Could you check a few things on this model? Use its own coordinates, in mm. A direction names the side the tool comes from. Give positions to 0.01 mm unless a question says otherwise; leave off trailing zeros. Order: outer loops, then holes, each group sorted by start corner. A loop starts at its lowest first (then second) coordinate and runs counter-clockwise, first axis right, second up.
from build123d import *

# Parameters (mm, degrees)
BOSS_EXTRUDE1_DEPTH = 100
CUT_EXTRUDE1_DEPTH  = 8
SKETCH4_W           = 8
SKETCH4_H           = 100
BOSS_EXTRUDE2_DEPTH = 35
CUT_EXTRUDE2_DEPTH  = 8


with BuildPart() as part:
    # Sketch1 → Boss-Extrude1 (new body)
    with BuildSketch(Plane(origin=(0, 0, 0), x_dir=(1, 0, 0), z_dir=(0, 1, 0))):
        Polygon((0, 0), (8, 0), (8, 27), (40, 27), (40, 35), (0, 35), align=None)
    extrude(amount=BOSS_EXTRUDE1_DEPTH)

    # Sketch3 → Cut-Extrude1 (cut)
    with BuildSketch(Plane(origin=(0, 0, -35), x_dir=(-1, 0, 0), z_dir=(0, 0, -1))):
        with BuildLine():
            Line((-40, 20), (-35, 20))
            ThreePointArc((-35, 20), (-31.464466094, 21.464466094), (-30, 25))
            Line((-30, 25), (-30, 75))
            ThreePointArc((-30, 75), (-31.464466094, 78.535533906), (-35, 80))
            Line((-35, 80), (-40, 80))
            Line((-40, 80), (-40, 20))
        make_face()
    extrude(amount=-CUT_EXTRUDE1_DEPTH, mode=Mode.SUBTRACT)

    # Sketch4 → Boss-Extrude2 (add)
    with BuildSketch(Plane(origin=(0, 0, -35), x_dir=(-1, 0, 0), z_dir=(0, 0, -1))):
        with Locations((-15, 50)):
            Rectangle(SKETCH4_W, SKETCH4_H)
    extrude(amount=BOSS_EXTRUDE2_DEPTH)

    # Sketch5 → Cut-Extrude2 (cut)
    with BuildSketch(Plane(origin=(19, 0, 0), x_dir=(0, 0, -1), z_dir=(1, 0, 0))):
        with BuildLine():
            Line((56, 86), (70, 86))
            Line((70, 86), (70, 74))
            Line((70, 74), (56, 74))
            ThreePointArc((56, 74), (50, 80), (56, 86))
        make_face()
        with BuildLine():
            Line((70, 54), (56, 54))
            ThreePointArc((56, 54), (50, 60), (56, 66))
            Line((56, 66), (70, 66))
            Line((70, 66), (70, 54))
        make_face()
        with BuildLine():
            Line((70, 34), (56, 34))
            ThreePointArc((56, 34), (50, 40), (56, 46))
            Line((56, 46), (70, 46))
            Line((70, 46), (70, 34))
        make_face()
        with BuildLine():
            Line((70, 14), (56, 14))
            ThreePointArc((56, 14), (50, 20), (56, 26))
            Line((56, 26), (70, 26))
            Line((70, 26), (70, 14))
        make_face()
    extrude(amount=-CUT_EXTRUDE2_DEPTH, mode=Mode.SUBTRACT)


solid = part.part
Item 1: Imagine slicing it at D-D on z = -32.5. List the corners of the cut face in (x, y) for me.
Findings:
outline: (0, 0) - (40, 0) - (40, 20) - (35, 20) arc R5 cw to (30, 25) - (30, 75) arc R5 cw to (35, 80) - (40, 80) - (40, 100) - (0, 100) - close
Item 2: For faces 1 (the flat face through (8, 49, -13)), 2 (the flat face through (15, 93, -70)), 3 (the flat face through (15, 46, -63)), 4 (the flat face through (11, 49, -48)), 5 (the flat face through (38, 20, -31)), which set-ups out of +Z, -Z, +X, -X, +Y, -Y let a thin tool reach every point of the face, with its end or its side?
Findings:
face 1: +Z, +X, +Y, -Y
face 2: -Z, +X, -X, +Y, -Y
face 3: -Z, +X, -X
face 4: -Z, -X, +Y, -Y
face 5: +Z, -Z, +X
Item 3: Please list where these lines run through material, in increasing order: line 1 along X through (y, z) = (80, -38.5); line 2 along Z through (x, y) = (9, 84); line 3 along X through (y, z) = (6.5, -5).
Findings:
line 1: x = 11 to 19
line 2: z = -35 to -27
line 3: x = 0 to 8
Item 4: Imagine slicing it at C-C on y = 48.5. List the corners of the cut face in (x, z) for me, then the cut area to 3 significant figures.
Findings:
outline: (0, -35) - (11, -35) - (11, -70) - (19, -70) - (19, -35) - (30, -35) - (30, -27) - (8, -27) - (8, 0) - (0, 0) - close
area: 736 mm2
Item 5: For pin 1 (8 mm diameter, centred on x = 27, y = 34.5, fed in from -Z); pin 2 (8 mm diameter, centred on y = 17, z = -45, fed in from +X); pin 3 (13.5 mm diameter, centred on y = 68.5, z = -12, fed in from +X), each with a flat end and sliding along its axis, tell me the tip position at first contact or that it passes through.
Findings:
pin 1: stops at z = -35
pin 2: stops at x = 19
pin 3: stops at x = 8
Item 6: Imagine slicing it at B-B on x = 32.5. List the corners of the cut face in (y, z) for me.
Findings:
outline: (0, -35) - (20.67, -35) - (20.67, -27) - (0, -27) - close; (79.33, -35) - (100, -35) - (100, -27) - (79.33, -27) - close
Item 7: Imagine slicing it at A-A on z = -65. List the corners of the cut face in (x, y) for me.
Findings:
outline: (11, 0) - (19, 0) - (19, 14) - (11, 14) - close; (11, 26) - (19, 26) - (19, 34) - (11, 34) - close; (11, 46) - (19, 46) - (19, 54) - (11, 54) - close; (11, 66) - (19, 66) - (19, 74) - (11, 74) - close; (11, 86) - (19, 86) - (19, 100) - (11, 100) - close
Item 8: We'd pull the mould along Y, two halves only. Please class faces 6 (the flat face through (6, 49, -35)), 7 (the flat face through (15, 54, -63)): +Y half, -Y half, draft (parallel to the pull), parting line (faces both ways), or undercut.
Findings:
face 6: draft
face 7: undercut
